The model under review builds one solid part; all positions refer to its coordinate system, in mm. A direction names the side the tool comes from. Round coordinates to 2 decimals unless told otherwise and drop trailing zeros. Order: outer loops, then holes, each group sorted by start corner. A loop starts at its lowest first (then second) coordinate and runs counter-clockwise, first axis right, second up.
1) Consider section A-A (y = 15.5). Give the boundary of the cut face in (x, z), then the cut area to 3 significant figures.
2) Mouldability with a two-part tool opening along X and no side actions: class faces 4 (the face through (15, 18, 42)), 5 (the face through (-2, 20, 48.051)), 6 (the face through (0, 22, 58.251)), 7 (the face through (6.466, 16.726, 39.4)) as pulls with the +X half, pulls with the -X half, needs draft (parallel to the pull), parting line crosses it, or undercut.
3) Clearance check with flat-ended pins moving along their axes: P1, Ø5, axis at x = -1, y = 17.5, coming from the -Z side; P2, Ø6, axis at x = 7.5, z = 38.05, coming from the +Y side; P3, Ø2, axis at x = 10, z = 52.15, coming from the +Y side. State where each tip first meets the part, or that it passes through.
4) Machinability: for faces 1 (the face through (-8.2, 16.7, 44.7)), 2 (the face through (0, 12.35, 29)), 3 (the face through (11.054, 21.19, 31.479)), which of the approach directions +Z, -Z, +X, -X, +Y, -Y give a long, thin tool a straight path to every point of the face, cutting with its end or side? Answer none if there is none.
5) Consider section C-C (z = 47). Give the boundary of the cut face in (x, y), then the cut area to 3 significant figures.
6) Consider section D-D (y = 13.75). Give the boundary of the cut face in (x, z), then the cut area to 3 significant figures.
7) To check wall thickness, follow L1, parallel to Z at x = 10, y = 22; L2, parallel to X at y = 22.5, z = 31.5; L3, parallel to X at y = 14.5, z = 39.5. State the ranges of each line that lie inside material, in increasing order.
8) Consider section B-B (x = -8). Give the boundary of the cut face in (y, z).
from build123d import *

# Parameters (mm, degrees)
SKETCH_1_W             = 30
SKETCH_1_H             = 32.2
BODY_DEPTH             = 14
FIXTURE_M3_D           = 3.4
FIXTURE_M3_DEPTH       = 14
FIXTURE_M3_CBORE_D     = 6.5
FIXTURE_M3_CBORE_DEPTH = 3.4
FIXTURE_M3_TIP         = 1.021463052
FIXTURE_M3_1_D         = 2.5
FIXTURE_M3_1_DEPTH     = 8.5
FIXTURE_M3_1_TIP       = 0.751075774
SKETCH_6_R             = 2.75
HOLE_DEPTH             = 32.2
OVAL_DEPTH             = 6
SKETCH_8_R             = 5
HOLE2_DEPTH            = 22


with BuildPart() as part:
    # Эскиз1 → Body (new body)
    with BuildSketch(Plane(origin=(0, 11.5, 0), x_dir=(1, 0, 0), z_dir=(0, 1, 0))):
        with Locations((0, -42.150641757)):
            Rectangle(SKETCH_1_W, SKETCH_1_H)
    extrude(amount=BODY_DEPTH)

    # Fixture M3
    with Locations(Plane(origin=(-7.5, 25.5, 38.050641757), x_dir=(0, 0, 1), z_dir=(0, 1, 0))):
        with Locations((0, 0), (8.2, 0), (0, 15), (8.2, 15)):
            CounterBoreHole(FIXTURE_M3_D / 2, FIXTURE_M3_CBORE_D / 2, FIXTURE_M3_CBORE_DEPTH, depth=FIXTURE_M3_DEPTH)
            with Locations((0, 0, -(FIXTURE_M3_DEPTH + FIXTURE_M3_TIP / 2))):  # 118° drill point
                Cone(0, FIXTURE_M3_D / 2, FIXTURE_M3_TIP, mode=Mode.SUBTRACT)

    # Fixture M3_1
    with Locations(Plane(origin=(-10, 25.5, 32.150641757), x_dir=(0, 0, 1), z_dir=(0, 1, 0))):
        with Locations((0, 0), (0, 20), (20, 20), (20, 0)):
            Hole(FIXTURE_M3_1_D / 2, depth=FIXTURE_M3_1_DEPTH)
            with Locations((0, 0, -(FIXTURE_M3_1_DEPTH + FIXTURE_M3_1_TIP / 2))):  # 118° drill point
                Cone(0, FIXTURE_M3_1_D / 2, FIXTURE_M3_1_TIP, mode=Mode.SUBTRACT)

    # Эскиз6 → Hole (cut)
    with BuildSketch(Plane.XY.offset(58.250641757)):
        with Locations((0, 17.35)):
            Circle(SKETCH_6_R)
    extrude(amount=-HOLE_DEPTH, mode=Mode.SUBTRACT)

    # Эскиз7 → Oval (cut)
    with BuildSketch(Plane(origin=(0, 0, 26.050641757), x_dir=(-1, 0, 0), z_dir=(0, 0, -1))):
        with BuildLine():
            Line((-2.5, 22.35), (2.5, 22.35))
            ThreePointArc((2.5, 22.35), (7.5, 17.35), (2.5, 12.35))
            Line((2.5, 12.35), (-2.5, 12.35))
            ThreePointArc((-2.5, 12.35), (-7.5, 17.35), (-2.5, 22.35))
        make_face()
    extrude(amount=-OVAL_DEPTH, mode=Mode.SUBTRACT)

    # Эскиз8 → Hole2 (cut)
    with BuildSketch(Plane(origin=(0, 0, 26.050641757), x_dir=(-1, 0, 0), z_dir=(0, 0, -1))):
        with Locations(Location((0, 17.35, 0), (0, 0, 90))):
            Circle(SKETCH_8_R)
    extrude(amount=-HOLE2_DEPTH, mode=Mode.SUBTRACT)


solid = part.part
Answer below:
1. outline: (-15, 26.05) - (-7.15, 26.05) - (-7.15, 32.05) - (-4.65, 32.05) - (-4.65, 48.05) - (-2.03, 48.05) - (-2.03, 58.25) - (-15, 58.25) - close; (2.03, 48.05) - (4.65, 48.05) - (4.65, 32.05) - (7.15, 32.05) - (7.15, 26.05) - (15, 26.05) - (15, 58.25) - (2.03, 58.25) - close; hole circle Ø3.4 at (-7.5, 38.05); hole circle Ø3.4 at (-7.5, 46.25); hole circle Ø3.4 at (7.5, 38.05); hole circle Ø3.4 at (7.5, 46.25)
1. area: 654 mm2
2. face 4: pulls with the +X half
2. face 5: undercut
2. face 6: needs draft
2. face 7: undercut
3. P1: stops at z = 48.05
3. P2: stops at y = 22.1
3. P3: stops at y = 16.85
4. face 1: +Y, -Y
4. face 2: -Z
4. face 3: +Y
5. outline: (-15, 11.5) - (-9.03, 11.5) - (-9.03, 22.1) - (-10.66, 22.1) - (-10.66, 25.5) - (-15, 25.5) - close; (-5.97, 11.5) - (5.97, 11.5) - (5.97, 22.1) - (4.34, 22.1) - (4.34, 25.5) - (-4.34, 25.5) - (-4.34, 22.1) - (-5.97, 22.1) - close; (9.03, 11.5) - (15, 11.5) - (15, 25.5) - (10.66, 25.5) - (10.66, 22.1) - (9.03, 22.1) - close; hole circle Ø10 at (0, 17.35)
5. area: 234 mm2
6. outline: (-15, 26.05) - (-5.97, 26.05) - (-5.97, 32.05) - (-3.47, 32.05) - (-3.47, 48.05) - (3.47, 48.05) - (3.47, 32.05) - (5.97, 32.05) - (5.97, 26.05) - (15, 26.05) - (15, 58.25) - (-15, 58.25) - close; hole circle Ø3.4 at (-7.5, 38.05); hole circle Ø3.4 at (-7.5, 46.25); hole circle Ø3.4 at (7.5, 38.05); hole circle Ø3.4 at (7.5, 46.25)
6. area: 747 mm2
7. L1: z = 26.05 to 30.9, 33.4 to 50.9, 53.4 to 58.25
7. L2: x = -15 to -11.07, -8.93 to 8.93, 11.07 to 15
7. L3: x = -15 to -8.39, -6.61 to -4.11, 4.11 to 6.61, 8.39 to 15
8. outline: (11.5, 26.05) - (25.5, 26.05) - (25.5, 34.84) - (22.1, 34.84) - (22.1, 36.43) - (11.5, 36.43) - close; (11.5, 39.68) - (22.1, 39.68) - (22.1, 41.26) - (25.5, 41.26) - (25.5, 43.04) - (22.1, 43.04) - (22.1, 44.63) - (11.5, 44.63) - close; (11.5, 47.88) - (22.1, 47.88) - (22.1, 49.46) - (25.5, 49.46) - (25.5, 58.25) - (11.5, 58.25) - close
